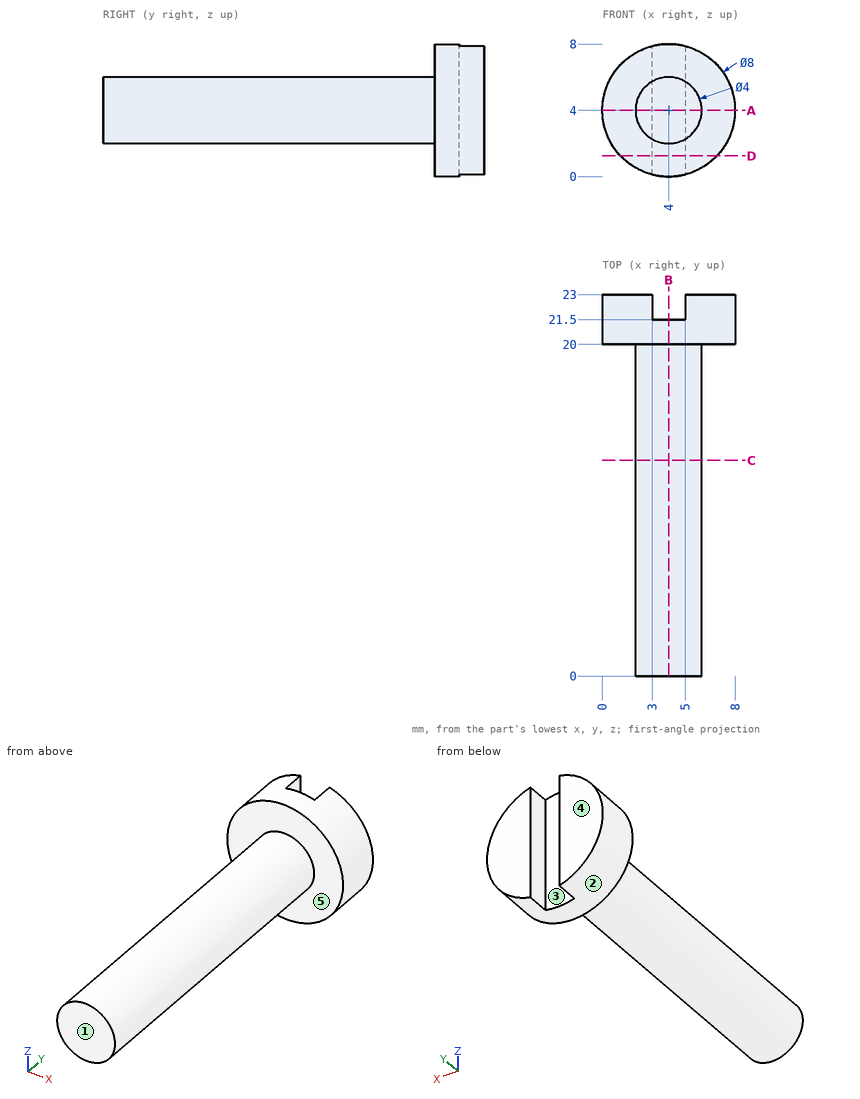
Answer from the drawing. Dimensions are ordinates in mm from the lowest x, y and z of the part. A direction names the side the tool comes from. Round coordinates to 2 decimals unless told otherwise and drop trailing zeros. Order: outer loops, then holes, each group sorted by start corner. A loop starts at its lowest first (then second) coordinate and runs counter-clockwise, first axis right, second up. Notation, with made-up numbers: (88, 22) - (140, 22) arc R23 cw to (140, 37) - close; hole circle Ø7 at (-36.5, 16). An arc over 180 degrees is marked (long way). Put each result on its own line as item: value. Start each with the question number.
(1) Determine the mould class of the marked faces 1, 2 and 3 for opening direction X: released by +X, released by -X, zero draft, split by the parting line, or undercut.
(2) For the marked faces 4 and 5, determine the directions among +Z, -Z, +X, -X, +Y, -Y from which every point of the face is accessible in a straight line to the end or side of a thin tool.
(3) Straight lines are drawn through the part: probe 1 along Y at (x, z) = (2.25, 2.75); probe 2 along Y at (x, z) = (4.25, 2.5); probe 3 along Z at (x, y) = (5.5, 12.25). For each, find the intervals that lie inside material, in ascending order. Write a range as from..to.
(4) Given P1, Ø1.5, axis at y = 12, z = 4, coming from the +X side; P2, Ø3, axis at x = 6.5, y = 4, coming from the +Z side; P3, Ø1.2, axis at y = 22.5, z = 2.5, coming from the -X side, each flat-ended and moving along its own axis, determine where each tip first touches the part or whether it passes through.
(5) Find section A-A (z = 4). Give the vertices of the cut face in (x, y).
(6) Find section B-B (x = 4). Give the vertices of the cut face in (y, z), plus the area to 3 significant figures.
(7) Find section C-C (y = 13). Give the vertices of the cut face in (x, z), plus the area to 3 significant figures.
(8) Find section D-D (z = 1.25). Give the vertices of the cut face in (x, y).
Reply:
1. face 1: zero draft
1. face 2: split by the parting line
1. face 3: undercut
2. face 4: +Z, -Z, +X, -X, +Y
2. face 5: -Y
3. probe 1: 20..23
3. probe 2: 0..21.5
3. probe 3: 2.68..5.32
4. P1: x = 6
4. P2: z = 5.73
4. P3: x = 0.1
5. outline: (0, 20) - (2, 20) - (2, 0) - (6, 0) - (6, 20) - (8, 20) - (8, 23) - (5, 23) - (5, 21.5) - (3, 21.5) - (3, 23) - (0, 23) - close
6. outline: (0, 2) - (20, 2) - (20, 0) - (21.5, 0) - (21.5, 8) - (20, 8) - (20, 6) - (0, 6) - close
6. area: 92.0 mm^2
7. outline: circle Ø4 at (4, 4)
7. area: 12.6 mm^2
8. outline: (1.1, 20) - (6.9, 20) - (6.9, 23) - (5, 23) - (5, 21.5) - (3, 21.5) - (3, 23) - (1.1, 23) - close
